The listing builds one solid part. Answer for the finished solid, in the listing's coordinates (mm). A direction names the side the tool comes from. Give positions to 0.01 mm unless a question says otherwise; leave off trailing zeros. Write each loop counter-clockwise with the first axis right and the second up, starting at its lowest first coordinate (ties: lowest second). Pieces come first, ordered by that corner, then holes. Notation, with made-up numbers: (77, -25) - (134, -25) arc R34 ccw to (134, 12) - close; hole circle Ø1 at (-17, 18). An arc over 180 degrees is marked (long way). Answer in a Markdown table with one row per item. Add a question column.
Autodesk Inventor part; units mm, degrees
ref_plane "YZ Plane" through (0, 0, 0) normal (1, 0, 0) x (0, 1, 0)
ref_plane "XZ Plane" through (0, 0, 0) normal (0, 1, 0) x (-1, 0, 0)
ref_plane "XY Plane" through (0, 0, 0) normal (0, 0, 1) x (1, 0, 0)
sketch "Sketch1" plane through (0, 0, 0) normal (1, 0, 0) x (0, 1, 0)
  line L0 (22.225, 22.225) -> (-22.225, 22.225)
  line L1 (-22.225, 22.225) -> (-22.225, -22.225)
  line L2 (-22.225, -22.225) -> (22.225, -22.225)
  line L3 (22.225, -22.225) -> (22.225, 22.225)
  line L4 (22.225, 22.225) -> (-22.225, -22.225) construction
  line L5 (-22.225, 22.225) -> (22.225, -22.225) construction
  point P0 (0, 0)
  dimension "d0" = 44.45
  dimension "d1" = 44.45
extrude "Extrusion1" add sketch "Sketch1" along normal blind 86.868
sketch "Sketch2" plane through (86.868, 0, 0) normal (1, 0, 0) x (0, 0, -1)
  circle A0 centre (0, 0) radius 28.956
  dimension "d4" = 57.912
extrude "Extrusion2" add sketch "Sketch2" along normal blind 58.166
sketch "Sketch3" plane through (0, 0, 0) normal (-1, 0, 0) x (0, 0, 1)
  circle A0 centre (0, 0) radius 6.35
  dimension "d7" = 12.7
extrude "Extrusion3" add sketch "Sketch3" along normal blind 139.7
equation "\"d1\" = d0"
properties part number "MotorAxel"
1. A tool of negligible diameter and unlimited length cuts with its end or side. For faces 1 (the face through (-68.87, 6.2, -1.38)), 2 (the face through (86.868, 25, 0)), 3 (the face through (43, 0, 22.225)), 4 (the face through (86.868, -25, 0)), 5 (the face through (43, 0, -22.225)), from which of +Z, -Z, +X, -X, +Y, -Y can it reach the whole face along a straight path? Write none if from no direction.
2. Section C-C (x = 125.5) is taken. Give the vertices of the cut face in (y, z), and give its area (3 significant figures).
3. Given pin 1 Ø1.1 at (y, z) = (-21, 21) entering from +X; pin 2 Ø2 at (x, y) = (28, 0.5) entering from +Z (3 decimals); pin 3 Ø6 at (x, z) = (-31, -7) entering from +Y, each flat-ended and moving along its own axis, determine where each tip first touches the part or whether it passes through.
4. Straight lines are drawn through the part: L1, parallel to Z at x = 79, y = 21.5 (3 decimals); L2, parallel to X at y = 11, z = -13.5. For each, find the intervals that lie inside material, in ascending order. Write a range as [from, to].
5. Section A-A (y = 0) is taken. Give the vertices of the cut face in (x, z) (3 decimals).
6. Section B-B (z = 12.5) is taken. Give the vertices of the cut face in (x, y) (3 decimals).
Geometry check:
| question | item | result |
|---|---|---|
| 1 | face 1 | -X |
| 1 | face 2 | +Z, -Z, -X, +Y |
| 1 | face 3 | +Z, -X, +Y, -Y |
| 1 | face 4 | +Z, -Z, -X, -Y |
| 1 | face 5 | -Z, -X, +Y, -Y |
| 2 | outline | circle Ø57.91 at (0, 0) |
| 2 | area | 2,630 mm² |
| 3 | pin 1 | x = 86.87 |
| 3 | pin 2 | z = 22.225 |
| 3 | pin 3 | y = 4.93 |
| 4 | L1 | [-22.225, 22.225] |
| 4 | L2 | [0, 145.03] |
| 5 | outline | (-139.7, -6.35) - (0, -6.35) - (0, -22.225) - (86.868, -22.225) - (86.868, -28.956) - (145.034, -28.956) - (145.034, 28.956) - (86.868, 28.956) - (86.868, 22.225) - (0, 22.225) - (0, 6.35) - (-139.7, 6.35) - close |
| 6 | outline | (0, -22.225) - (86.868, -22.225) - (86.868, -26.119) - (145.034, -26.119) - (145.034, 26.119) - (86.868, 26.119) - (86.868, 22.225) - (0, 22.225) - close |
